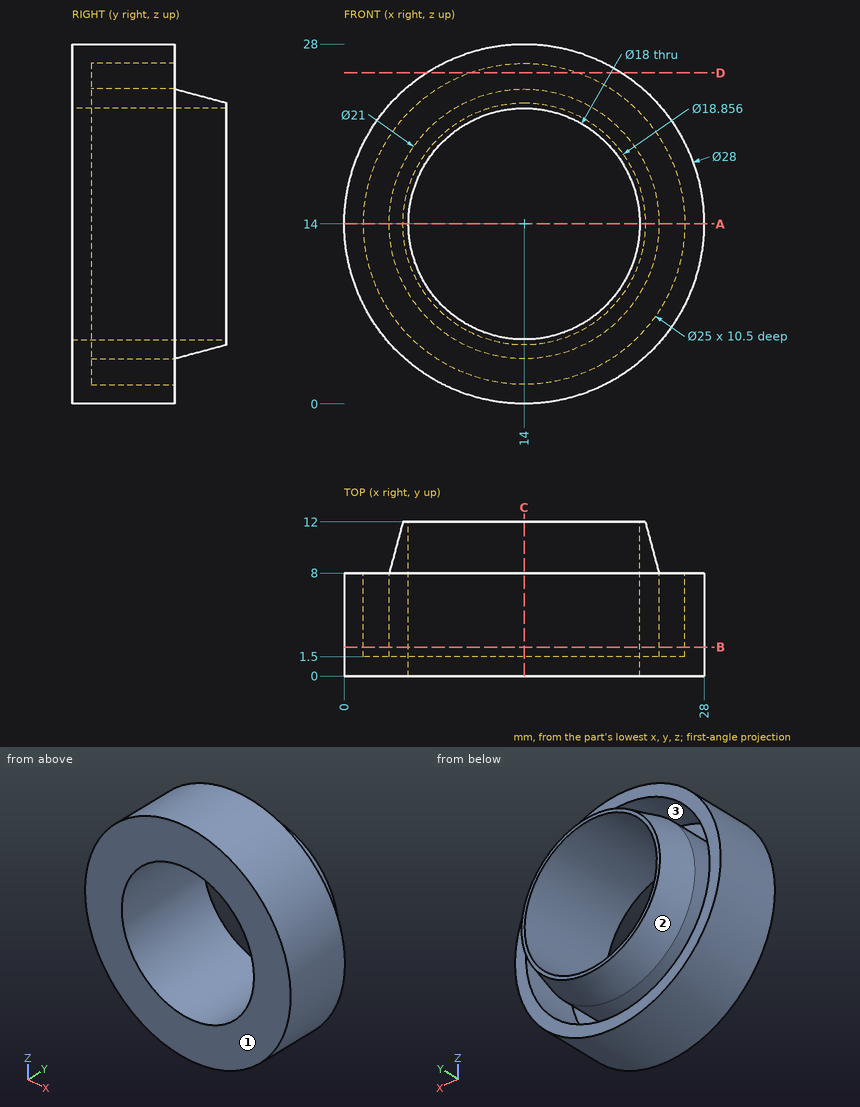
The drawing under review shows one solid part. Ordinate dimensions are in mm from its lowest x, y, z. Coordinates: 2 decimals unless noted, no trailing zeros. Write each loop counter-clockwise with the first axis right and the second up, starting at its lowest first coordinate (ties: lowest second). Pieces come first, ordered by that corner, then holes. Notation, with made-up numbers: (80, 14) -> (131, 14) arc R16 ccw to (131, 44) -> close; hole circle Ø9 at (24.25, -9). An arc over 180 degrees is marked (long way). Write each question's results on one line, items separated by ' | '. Start each with the question number.
1) The part is to be moulded in two halves that separate along X. For the marked faces 1, 2 and 3, say which applies: +X half, -X half, draft (parallel to the pull), parting line (faces both ways), or undercut.
2) Consider section B-B (y = 2.25). Write out the cut boundary in (x, z), plus the area to 3 significant figures.
3) Consider section A-A (z = 14). Write out the cut boundary in (x, y).
4) Wall thickness on L1, parallel to X at y = 4.5, z = 14; L2, parallel to Z at x = 20.5, y = 6.5 (1 decimal); L3, parallel to Z at x = 17.5, y = 7.75 (1 decimal): over which ranges is each line inside the solid? List them lowest first. Write a range as [from, to].
5) Consider section D-D (z = 25.75). Write out the cut boundary in (x, y) (1 decimal).
6) Insertion check: pin 1 (2 mm diameter, centred on y = 6.5, z = 18.5, fed in from +X) (1 decimal); pin 2 (8.5 mm diameter, centred on x = 16, z = 15, fed in from +Y); pin 3 (1.5 mm diameter, centred on y = 8, z = 9.5, fed in from -X); pin 4 (6 mm diameter, centred on y = 2.5, z = 25, fed in from +X). Each pin has a flat end and moves straight along its axis. Give the tip position at first contact, or say it passes through.
7) Consider section C-C (x = 14). Write out the cut boundary in (y, z).
Geometry says:
1) face 1: draft | face 2: parting line | face 3: undercut
2) outline: circle Ø28 at (14, 14); circle Ø21 at (14, 14); hole circle Ø25 at (14, 14); hole circle Ø18 at (14, 14) | area: 217 mm^2
3) outline: (0, 0) -> (5, 0) -> (5, 12) -> (4.57, 12) -> (3.5, 8) -> (3.5, 1.5) -> (1.5, 1.5) -> (1.5, 8) -> (0, 8) -> close; (23, 0) -> (28, 0) -> (28, 8) -> (26.5, 8) -> (26.5, 1.5) -> (24.5, 1.5) -> (24.5, 8) -> (23.43, 12) -> (23, 12) -> close
4) L1: [0, 1.5], [3.5, 5], [23, 24.5], [26.5, 28] | L2: [1.6, 3.3], [5.8, 7.8], [20.2, 22.2], [24.7, 26.4] | L3: [0.4, 2], [4.1, 5.7], [22.3, 23.9], [26, 27.6]
5) outline: (6.4, 0) -> (21.6, 0) -> (21.6, 8) -> (18.3, 8) -> (18.3, 1.5) -> (9.7, 1.5) -> (9.7, 8) -> (6.4, 8) -> close
6) pin 1: x = 27.6 | pin 2: through | pin 3: x = 0.51 | pin 4: x = 25.49
7) outline: (0, 0) -> (8, 0) -> (8, 1.5) -> (1.5, 1.5) -> (1.5, 3.5) -> (8, 3.5) -> (12, 4.57) -> (12, 5) -> (0, 5) -> close; (0, 23) -> (12, 23) -> (12, 23.43) -> (8, 24.5) -> (1.5, 24.5) -> (1.5, 26.5) -> (8, 26.5) -> (8, 28) -> (0, 28) -> close
